from build123d import *

# Parameters (mm, degrees)
SKETCH2_W           = 5
SKETCH2_H           = 53.8
BOSS_EXTRUDE1_DEPTH = 36
CUT_EXTRUDE1_DEPTH  = 15.943798685
SKETCH4_R           = 2.1
SKETCH4_R_2         = 4
CUT_EXTRUDE2_DEPTH  = 6


with BuildPart() as part:
    # Sketch2 → Boss-Extrude1 (new body)
    with BuildSketch(Plane(origin=(0, 629.439859668, -2204.462438001), x_dir=(1, 0, 0), z_dir=(0, -0.274557173, 0.961570777))):
        with Locations((-194.323635178, 2543.140113693)):
            Rectangle(SKETCH2_W, SKETCH2_H)
    extrude(amount=BOSS_EXTRUDE1_DEPTH)

    # Sketch3 → Cut-Extrude1 (cut, through all)
    with BuildSketch(Plane(origin=(67.333864744, -30.465363781, -80.619122615), x_dir=(0.491076421, 0.867206701, 0.082440809), z_dir=(0.615661475, -0.278557467, -0.737134103))):
        Polygon((2395.145764251, -2402.321354937), (2500.725824186, -2486.45131954), (2658.658473348, -2288.251562261), (2553.078413412, -2204.121597658), align=None)
    extrude(amount=-CUT_EXTRUDE1_DEPTH, mode=Mode.SUBTRACT)

    # Sketch4 → Cut-Extrude2 (cut, through all)
    with BuildSketch(Plane.ZY.offset(196.823635178)):
        with Locations((-1506.592316509, 3053.530651846)):
            Circle(SKETCH4_R)
        with Locations((-1482.553047089, 3046.666722522)):
            Circle(SKETCH4_R)
        with Locations((-1499.728387186, 3077.569921266)):
            Circle(SKETCH4_R)
        with Locations((-1475.689117766, 3070.705991942)):
            Circle(SKETCH4_R)
        with Locations((-1470.88436724, 3087.533480536)):
            Circle(SKETCH4_R)
        with Locations((-1494.92363666, 3094.397409859)):
            Circle(SKETCH4_R)
        with Locations((-1484.276787814, 3086.157591314)):
            Circle(SKETCH4_R_2)
        with Locations((-1491.140717138, 3062.118321894)):
            Circle(SKETCH4_R_2)
    extrude(amount=-CUT_EXTRUDE2_DEPTH, mode=Mode.SUBTRACT)


solid = part.part
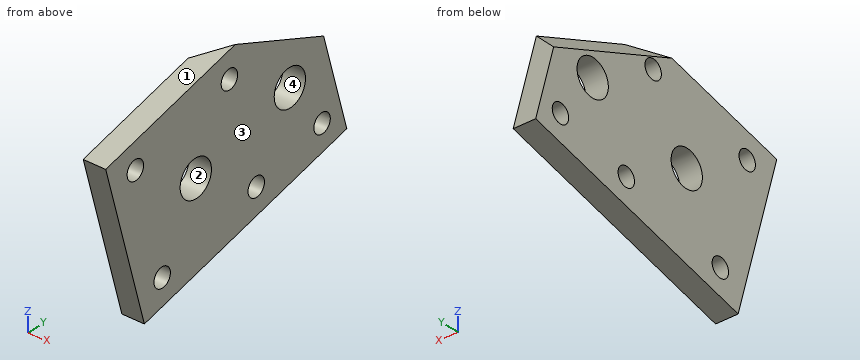
Can you work these out from the model? Positions are in its coordinate system, mm. Face numbers are marked on the shaded views. Round coordinates to 2 decimals unless told otherwise and drop trailing zeros. Loops run counter-clockwise (first coordinate to the right, second up) from the corner with the lowest first, then second, coordinate; pieces in that order, holes last. Notation, with made-up numbers: (6, 19) - (19, 19) arc R27 ccw to (19, 40) - close; hole circle Ø11 at (57.25, -20). An arc over 180 degrees is marked (long way). Write item = value, one per line. Start each with the question number.
(1) If we section it at D-D (y = 3095.5): Please give me the cut outline in (x, z).
(2) If we section it at A-A (z = -1506): Please give me the cut outline in (x, y).
(3) If we section it at C-C (x = -195.35): Please give me the cut outline in (y, z), and give its area (3 significant figures).
(4) If we section it at B-B (y = 3087): Please give me the cut outline in (x, z), and give its area (3 significant figures).
(5) For P1, Ø1, axis at x = -194, y = 3087, coming from the -Z side, with a flat end and sliding along its axis, tell me the tip position at first contact or that it passes through.
(6) If I drill on probe 1 along Y at (x, z) = (-195.4, -1493); probe 2 along Z at (x, y) = (-192.35, 3082.5); probe 3 along Z at (x, y) = (-192.75, 3084.5), over which ranges is the centre line in solid material (lowest first)? Write a range as [from, to].
(7) If we mould it in two halves opening along Z, with no side actions, what happens to the marked faces 1, 2, 3 and 4? For each: released by +Z, released by -Z, zero draft, split by the parting line, or undercut.
Ans:
q1.outline = (-196.82, -1500.33) - (-191.82, -1500.33) - (-191.82, -1496.71) - (-196.82, -1496.71) - close; (-196.82, -1493.14) - (-191.82, -1493.14) - (-191.82, -1480.57) - (-194.49, -1480.57) - (-196.82, -1482.52) - close
q2.outline = (-196.82, 3046.81) - (-191.82, 3046.81) - (-191.82, 3051.52) - (-196.82, 3051.52) - close; (-196.82, 3055.55) - (-191.82, 3055.55) - (-191.82, 3075.64) - (-196.82, 3075.64) - close
q3.outline = (3039.1, -1478.99) - (3048.98, -1513.61) - (3100.72, -1498.84) - (3095.73, -1481.38) - (3067.76, -1470.81) - close; hole circle Ø4.2 at (3046.67, -1482.55); hole circle Ø4.2 at (3053.53, -1506.59); hole circle Ø8 at (3062.12, -1491.14); hole circle Ø4.2 at (3070.71, -1475.69); hole circle Ø4.2 at (3077.57, -1499.73); hole circle Ø8 at (3086.16, -1484.28); hole circle Ø4.2 at (3094.4, -1494.92)
q3.area = 1,550 mm²
q4.outline = (-196.82, -1502.76) - (-191.82, -1502.76) - (-191.82, -1488.19) - (-196.82, -1488.19) - close; (-196.82, -1480.37) - (-191.82, -1480.37) - (-191.82, -1475.14) - (-196.82, -1479.31) - close
q4.area = 88.6 mm²
q5.P1 = -1502.9
q6.probe_1 = [3043.1, 3058.58], [3065.66, 3093.56], [3095.24, 3099.05]
q6.probe_2 = [-1504.04, -1485.9], [-1482.66, -1473.88]
q6.probe_3 = [-1503.47, -1487.92], [-1480.64, -1474.97]
q7.face_1 = released by +Z
q7.face_2 = undercut
q7.face_3 = zero draft
q7.face_4 = undercut
